Can you work these out from the model? Positions are in its coordinate system, mm. Face numbers are marked on the shaded views. A direction names the side the tool comes from. Coordinates: 2 decimals unless noted, no trailing zeros. Loops run counter-clockwise (first coordinate to the right, second up) from the corner with the lowest first, then second, coordinate; pieces in that order, holes last. Notation, with made-up numbers: M 26.5,-28.5 L 42.5,-28.5 A36 ccw 42.5,7.5 Z; hole C 67,-20 d6. An arc over 180 degrees is marked long. Answer as a JSON object with one key per item and string values. Group by question number.
Item 1: If I drill on line 1 (Y direction, x = 55, z = 8); line 2 (Y direction, x = 0, z = 15.5); line 3 (X direction, y = -1, z = 28), over which ranges is the centre line in solid material (lowest first)?
Item 2: Suppose I cut it at C-C (y = 8). Write out the boundary of the cut face in (x, z).
Item 3: Suppose I cut it at B-B (z = 16.5). Write out the boundary of the cut face in (x, y) (3 decimals), then the cut area to 3 significant figures.
Item 4: Suppose I cut it at A-A (x = 0). Write out the boundary of the cut face in (y, z).
Item 5: I'm going to push flat-ended pins straight in: pin 1 Ø12 at (x, z) = (12, 32.5) entering from -Y; pin 2 Ø10 at (x, z) = (-37, 5.5) entering from +Y; pin 3 Ø6 at (y, z) = (-9.5, 32.5) entering from +X; pin 4 Ø23 at (x, y) = (0, 0) entering from -Z. Where does each tip first touch, or does it pass through?
Item 6: Which directions (+Z, -Z, +X, -X, +Y, -Y) give clear straight access to the entire face, cutting with the end or side of a thin tool? Please do the marked faces 1, 2 and 3.
Item 7: Suppose I cut it at D-D (z = 29). Write out the boundary of the cut face in (x, y).
Item 8: We'd pull the mould along Y, two halves only. Please class the marked faces 4, 5 and 6: +Y half, -Y half, draft (parallel to the pull), parting line (faces both ways), or undercut.
```python
from build123d import *

# Parameters (mm, degrees)
F0_R     = 19.05
F1_DEPTH = 50.8
F0_R_2   = 9.525
F2_DEPTH = 19.05
F3_DEPTH = 19.05


with BuildPart() as f1:
    # F0 (on Top) → F1 (new body)
    with BuildSketch(Plane.XY):
        with BuildLine():
            ThreePointArc((29.147548, -12.589001), (31.092581, -6.427591), (31.75, 0))
            ThreePointArc((31.75, 0), (31.098159, 6.400547), (29.169401, 12.538283))
            ThreePointArc((29.169401, 12.538283), (0.010397, 31.749998), (-29.161183, 12.557384))
            ThreePointArc((-29.161183, 12.557384), (-31.749993, -0.021323), (-29.14429, -12.596541))
            ThreePointArc((-29.14429, -12.596541), (0.004107, -31.75), (29.147548, -12.589001))
        make_face()
        Circle(F0_R, mode=Mode.SUBTRACT)
    extrude(amount=F1_DEPTH)

    # F0 (on Top) → F2 (join)
    with BuildSketch(Plane.XY):
        with BuildLine():
            ThreePointArc((-29.14429, -12.596541), (-31.749993, -0.021323), (-29.161183, 12.557384))
            Line((-29.161183, 12.557384), (-48.945453, 12.563863))
            ThreePointArc((-48.945453, 12.563863), (-63.499337, 0.129762), (-49.202569, -12.599135))
            Line((-49.202569, -12.599135), (-29.14429, -12.596541))
        make_face()
        with Locations((-44.845603, 0)):
            Circle(F0_R_2, mode=Mode.SUBTRACT)
    extrude(amount=F2_DEPTH)

    # F0 (on Top) → F3 (join)
    with BuildSketch(Plane.XY):
        with BuildLine():
            ThreePointArc((29.169401, 12.538283), (31.098159, 6.400547), (31.75, 0))
            ThreePointArc((31.75, 0), (31.092581, -6.427591), (29.147548, -12.589001))
            Line((29.147548, -12.589001), (67.717979, -12.584012))
            ThreePointArc((67.717979, -12.584012), (79.23174, -0.579906), (68.988677, 12.525243))
            Line((68.988677, 12.525243), (29.169401, 12.538283))
        make_face()
        with BuildLine():
            ThreePointArc((67.717979, -9.390889), (66.604114, -9.462856), (65.489479, -9.404025))
            Line((65.489479, -9.404025), (45.251264, -9.523317))
            ThreePointArc((45.251264, -9.523317), (35.54757, -0.081586), (45.088101, 9.524987))
            Line((45.088101, 9.524987), (66.520438, 9.586939))
            ThreePointArc((66.520438, 9.586939), (76.054064, 0.661833), (67.717979, -9.390889))
        make_face(mode=Mode.SUBTRACT)
    extrude(amount=F3_DEPTH)


solid = f1.part
```
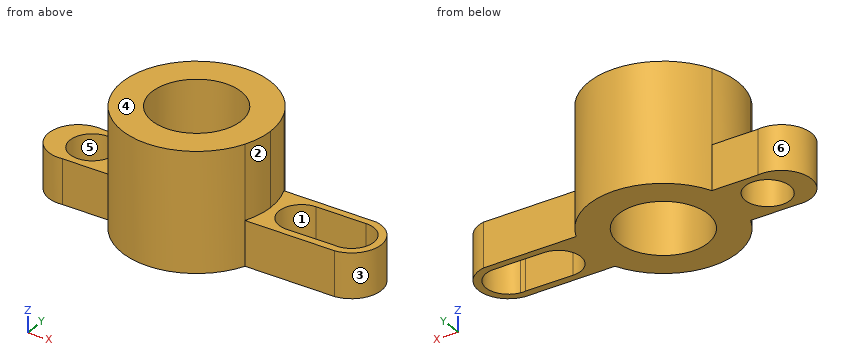
From the geometry:
{
 "1": {"line 1": "-12.59 to -9.47, 9.55 to 12.53", "line 2": "-31.75 to -19.05, 19.05 to 31.75", "line 3": "-31.73 to -19.02, 19.02 to 31.73"},
 "2": {"outline": "M -60.66,0 L -50.02,0 L -50.02,19.05 L -60.66,19.05 Z; M -39.68,0 L -17.29,0 L -17.29,50.8 L -30.73,50.8 L -30.73,19.05 L -39.68,19.05 Z; M 17.29,0 L 39.9,0 L 39.9,19.05 L 30.73,19.05 L 30.73,50.8 L 17.29,50.8 Z; M 71.81,0 L 76.46,0 L 76.46,19.05 L 71.81,19.05 Z"},
 "3": {"outline": "M -49.203,-12.599 L -29.144,-12.597 A31.75 ccw 29.148,-12.589 L 67.718,-12.584 A12.7 ccw 68.989,12.525 L 29.169,12.538 A31.75 ccw -29.161,12.557 L -48.945,12.564 A12.7 ccw long Z; hole C -44.846,0 d19.05; hole C 0,0 d38.1; hole M 45.088,9.525 A9.525 ccw long 45.251,-9.523 L 65.489,-9.404 A9.525 ccw 67.718,-9.391 A9.525 ccw 66.52,9.587 Z", "area": "2,950 mm2"},
 "4": {"outline": "M -31.75,0 L -19.05,0 L -19.05,50.8 L -31.75,50.8 Z; M 19.05,0 L 31.75,0 L 31.75,50.8 L 19.05,50.8 Z"},
 "5": {"pin 1": "y = -31.18", "pin 2": "y = 12.56", "pin 3": "x = 31.08", "pin 4": "through"},
 "6": {"face 1": "+Z, -Z", "face 2": "+Z, +X, -Y", "face 3": "+Z, -Z, +X"},
 "7": {"outline": "M -29.16,12.56 A31.75 ccw -29.14,-12.6 A31.75 ccw 29.15,-12.59 A31.75 ccw 31.75,0 A31.75 ccw 29.17,12.54 A31.75 ccw Z; hole C 0,0 d38.1"},
 "8": {"face 4": "draft", "face 5": "undercut", "face 6": "parting line"}
}
